Geometry: see drawing. Coordinates: mm, zero at the bounding-box minimum. Give positions to 0.01 mm unless a question says otherwise; leave off trailing zeros. Write each loop counter-clockwise with the first axis right and the second up, starting at its lowest first coordinate (ties: lowest second). Pieces come first, ordered by that corner, then holes. Notation, with made-up numbers: (61, 15) -> (84, 15) arc R15 cw to (84, 43) -> close; hole circle Ø3 at (-5, 32.25). An arc over 180 degrees is marked (long way). Answer as a JSON object with one key per item and string values. Group by question number.
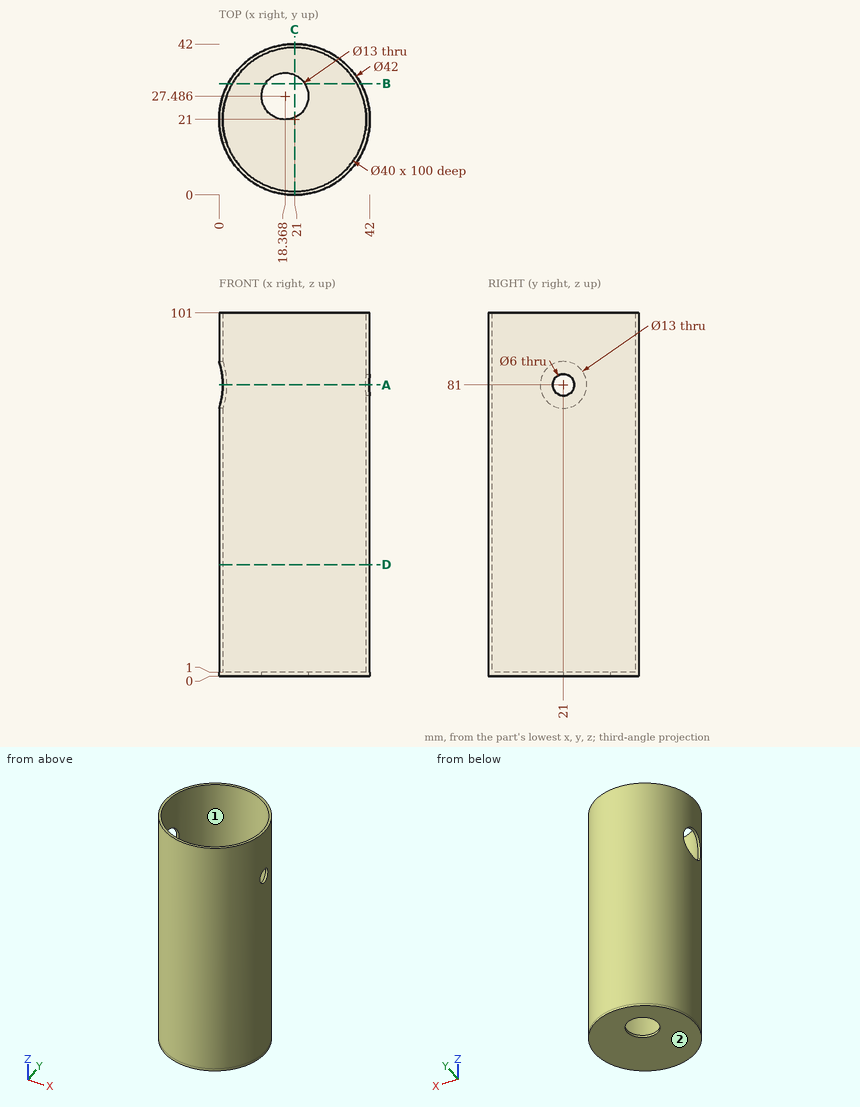
1. Section A-A (z = 81). Return the cut outline in (x, y) (1 decimal).
2. Section D-D (z = 31). Return the cut outline in (x, y), plus the area to 3 significant figures.
3. Section C-C (x = 21). Return the cut outline in (y, z).
4. Line query: line 1 (Y direction, x = 20.5, z = 28); line 2 (Z direction, x = 31, y = 11). Output: solid intervals per line, ascending.
5. Section B-B (y = 31). Return the cut outline in (x, z).
6. Contact query for flat-ended pins moving along their axis: pin 1 Ø6 at (x, z) = (19, 85.5) entering from -Y; pin 2 Ø8 at (x, y) = (18.37, 27.49) entering from -Z; pin 3 Ø5 at (y, z) = (26.5, 50) entering from +X (1 decimal); pin 4 Ø7 at (y, z) = (21, 81) entering from -X. Output: stop coordinate, or through.
7. Mould query, pull axis Y, two halves, no side actions, for the marked faces 1 and 2. Classes: pulls with the +Y half, pulls with the -Y half, needs draft (parallel to the pull), parting line crosses it, or undercut.
Working result:
{
 "1": {"outline": "(1, 14.5) arc R21 ccw to (41.8, 18) -> (40.8, 18) arc R20 cw to (2.1, 14.5) -> close; (1, 27.5) -> (2.1, 27.5) arc R20 cw to (40.8, 24) -> (41.8, 24) arc R21 ccw to start"},
 "2": {"outline": "circle Ø42 at (21, 21); hole circle Ø40 at (21, 21)", "area": "129 mm^2"},
 "3": {"outline": "(0, 0) -> (21.54, 0) -> (21.54, 1) -> (1, 1) -> (1, 101) -> (0, 101) -> close; (33.43, 0) -> (42, 0) -> (42, 101) -> (41, 101) -> (41, 1) -> (33.43, 1) -> close"},
 "4": {"line 1": "y = 0.01 to 1.01, 40.99 to 41.99", "line 2": "z = 0 to 1"},
 "5": {"outline": "(2.53, 0) -> (12.9, 0) -> (12.9, 1) -> (3.68, 1) -> (3.68, 101) -> (2.53, 101) -> close; (23.84, 0) -> (39.47, 0) -> (39.47, 101) -> (38.32, 101) -> (38.32, 1) -> (23.84, 1) -> close"},
 "6": {"pin 1": "stops at y = 0", "pin 2": "passes through", "pin 3": "stops at x = 41.8", "pin 4": "stops at x = 40.69"},
 "7": {"face 1": "undercut", "face 2": "needs draft"}
}
